Work out the finished part from the listing and answer in its coordinate system (mm). Face numbers are marked on the shaded views. A direction names the side the tool comes from. Give positions to 0.01 mm unless a question says otherwise; leave off trailing zeros. Loops run counter-clockwise (first coordinate to the right, second up) from the corner with the lowest first, then second, coordinate; pieces in that order, holes last. Notation, with made-up numbers: (35.25, 81) - (56.25, 81) arc R12 ccw to (56.25, 86) - close; hole circle Ø2 at (-8, 43). An arc over 180 degrees is marked (long way). One line per item, written item: value.
from build123d import *

# Parameters (mm, degrees)
F0_W     = 1.6002
F0_H     = 1.57988
F0_H_2   = 1.59004
F0_W_2   = 12.7
F0_H_3   = 1.6002
F1_DEPTH = 3.175
F2_T     = -1.6002
F3_DEPTH = 25.4
F4_W     = 1.6002
F4_H     = 1.59004
F4_H_2   = 1.57988
F5_DEPTH = 1.6002


with BuildPart() as f1:
    # F0 (on Top) → F1 (new body)
    with BuildSketch(Plane.XY):
        with Locations((8.509001, -9.207606)):
            Rectangle(F0_W, F0_H)
        with Locations((-5.791199, -4.442566)):
            Rectangle(F0_W, F0_H_2)
        with Locations((8.509001, -4.442566)):
            Rectangle(F0_W, F0_H_2)
        with Locations((1.358901, -4.442566)):
            Rectangle(F0_W_2, F0_H_2)
        with Locations((1.358901, -7.622646)):
            Rectangle(F0_W_2, F0_H_2)
        with Locations((-5.791199, -10.797646)):
            Rectangle(F0_W, F0_H_3)
        with Locations((-5.791199, -6.032606)):
            Rectangle(F0_W, F0_H_2)
        with Locations((-5.791199, -7.622646)):
            Rectangle(F0_W, F0_H_2)
        with Locations((-5.791199, -9.207606)):
            Rectangle(F0_W, F0_H)
        with Locations((8.509001, -6.032606)):
            Rectangle(F0_W, F0_H_2)
        with Locations((8.509001, -7.622646)):
            Rectangle(F0_W, F0_H_2)
        with Locations((8.509001, -10.797646)):
            Rectangle(F0_W, F0_H_3)
        with Locations((1.358901, -6.032606)):
            Rectangle(F0_W_2, F0_H_2)
        with Locations((1.358901, -9.207606)):
            Rectangle(F0_W_2, F0_H)
        with Locations((1.358901, -10.797646)):
            Rectangle(F0_W_2, F0_H_3)
    extrude(amount=F1_DEPTH)

    # F2
    f2_openings = [f1.faces().sort_by_distance(p)[0] for p in [
        (1.358901, -7.622646, 0),
    ]]
    offset(amount=F2_T, openings=f2_openings)

    # F0 (on Top) → F3 (cut)
    with BuildSketch(Plane.XY):
        with Locations((1.358901, -6.032606)):
            Rectangle(F0_W_2, F0_H_2)
        with Locations((1.358901, -9.207606)):
            Rectangle(F0_W_2, F0_H)
    extrude(amount=F3_DEPTH, mode=Mode.SUBTRACT)

    # F4 (on face) → F5 (cut)
    with BuildSketch(Plane.XY.offset(3.175)):
        with Locations((-5.791199, -6.032606)):
            Rectangle(F4_W, F4_H)
        with Locations((-5.791199, -9.207606)):
            Rectangle(F4_W, F4_H_2)
        with Locations((8.509001, -6.032606)):
            Rectangle(F4_W, F4_H)
        with Locations((8.509001, -9.207606)):
            Rectangle(F4_W, F4_H_2)
    extrude(amount=-F5_DEPTH, mode=Mode.SUBTRACT)


solid = f1.part
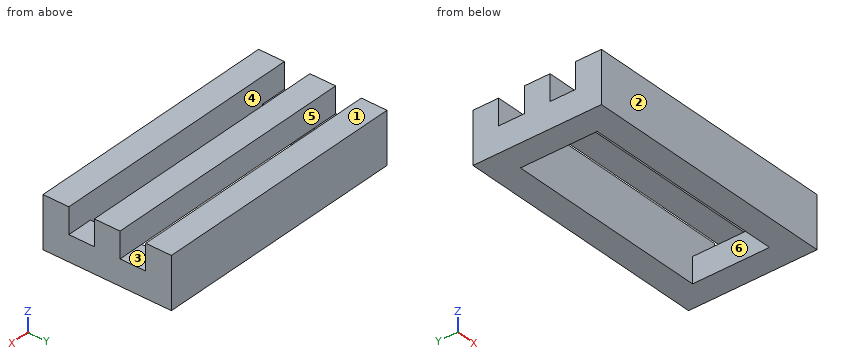
1. Section B-B (y = -6) is taken. Write down the section's boundary in (x, z), and give its area (3 significant figures).
Output:
outline: (-6.59, 0) - (-4.99, 0) - (-4.99, 1.57) - (-6.59, 1.57) - close; (7.71, 0) - (9.31, 0) - (9.31, 1.57) - (7.71, 1.57) - close
area: 5.04 mm²
2. For the marked faces 4, 5 and 6, determine the directions among +Z, -Z, +X, -X, +Y, -Y from which every point of the face is accessible in a straight line to the end or side of a thin tool.
Output:
face 4: +Z
face 5: +Z, +X, -X
face 6: -Z
3. Find the intervals of material crossed by line 1 along Y through (x, z) = (2.25, 2.95); line 2 along Y through (x, z) = (2.25, 1.3); line 3 along X through (y, z) = (-8, 1.05), in increasing order.
Output:
line 1: y = -11.6 to -10, -8.42 to -6.83, -5.24 to -3.65
line 2: y = -11.6 to -10, -5.24 to -3.65
line 3: x = -6.59 to -4.99, 7.71 to 9.31
4. The mould has two halves that part along Y. Classify the marked faces 1, 2 and 3: released by +Y, released by -Y, zero draft, split by the parting line, or undercut.
Output:
face 1: zero draft
face 2: released by -Y
face 3: undercut
5. Section D-D (z = 2.6) is taken. Write down the section's boundary in (x, y).
Output:
outline: (-6.59, -11.6) - (9.31, -11.6) - (9.31, -10) - (-6.59, -10) - close; (-6.59, -8.42) - (9.31, -8.42) - (9.31, -6.83) - (-6.59, -6.83) - close; (-6.59, -5.24) - (9.31, -5.24) - (9.31, -3.65) - (-6.59, -3.65) - close
6. Section A-A (x = 6.5) is taken. Write down the section's boundary in (y, z) (3 decimals), and give its area (3 significant figures).
Output:
outline: (-11.598, 0) - (-9.998, 0) - (-9.998, 3.175) - (-11.598, 3.175) - close; (-8.418, 1.575) - (-6.828, 1.575) - (-6.828, 3.175) - (-8.418, 3.175) - close; (-5.238, 0) - (-3.648, 0) - (-3.648, 3.175) - (-5.238, 3.175) - close
area: 12.7 mm²
7. Flat-ended cylindrical pins translate along their axes: pin 1 Ø0.8 at (x, y) = (-5.5, -9.5) entering from +Z; pin 2 Ø0.5 at (x, y) = (-1, -7.5) entering from -Z. Find the tip coordinate at first contact, or state that the pin passes through.
Output:
pin 1: stops at z = 1.57
pin 2: stops at z = 1.57
8. Section C-C (z = 0.4) is taken. Write down the section's boundary in (x, y).
Output:
outline: (-6.59, -11.6) - (9.31, -11.6) - (9.31, -3.65) - (-6.59, -3.65) - close; hole (-4.99, -10) - (7.71, -10) - (7.71, -5.24) - (-4.99, -5.24) - close
